from build123d import *

# Parameters (mm, degrees)
BASE_EXTRUDE_DEPTH = 11.1125
SKETCH2_R          = 4.1656
HOLE1_DEPTH        = 39.1
SKETCH3_R          = 3.2639
HOLE2_DEPTH        = 39.1


with BuildPart() as part:
    # Sketch1 → Base Extrude (new body, symmetric)
    with BuildSketch(Plane(origin=(0, 0, 0), x_dir=(0, 0, -1), z_dir=(1, 0, 0))):
        with BuildLine():
            Line((-4.7752, 9.5504), (-4.7752, 33.3248))
            ThreePointArc((-4.7752, 33.3248), (-3.376576302, 36.701376302), (0, 38.1))
            Line((0, 38.1), (0, 0))
            Line((0, 0), (-38.1, 0))
            ThreePointArc((-38.1, 0), (-36.701376302, 3.376576302), (-33.3248, 4.7752))
            Line((-33.3248, 4.7752), (-9.5504, 4.7752))
            ThreePointArc((-9.5504, 4.7752), (-6.173823698, 6.173823698), (-4.7752, 9.5504))
        make_face()
    extrude(amount=BASE_EXTRUDE_DEPTH, both=True)

    # Sketch2 → Hole1 (cut, through all)
    with BuildSketch(Plane.XZ):
        with Locations((0, 19.05)):
            Circle(SKETCH2_R)
    extrude(amount=-HOLE1_DEPTH, mode=Mode.SUBTRACT)

    # Sketch3 → Hole2 (cut, through all)
    with BuildSketch(Plane(origin=(0, 0, 0), x_dir=(-1, 0, 0), z_dir=(0, 0, -1))):
        with Locations((0, 19.05)):
            Circle(SKETCH3_R)
    extrude(amount=-HOLE2_DEPTH, mode=Mode.SUBTRACT)


solid = part.part
Geometry check sheet. Reference: the model listing, model coordinates, mm. A direction names the side the tool comes from. Give positions to 0.01 mm unless a question says otherwise; leave off trailing zeros. Write each loop counter-clockwise with the first axis right and the second up, starting at its lowest first coordinate (ties: lowest second). Pieces come first, ordered by that corner, then holes. Notation, with made-up numbers: M 88.5,30 L 93.5,30 A13 ccw 93.5,45 Z; hole C 46,-22.75 d4. An arc over 180 degrees is marked long. Answer as CSV lines item,"result". Start each with the question number.
Q1. Section check C-C, the plane z = 19.05. Record the cut outline in (x, y), then the cut area to 3 significant figures.
Q2. Section check B-B, the plane x = 0. Record the cut outline in (y, z).
Q3. Material ranges on L1, parallel to X at y = 2, z = 19; L2, parallel to X at y = 19, z = 3; L3, parallel to Y at x = 3.75, z = 24, recorded low to high.
Q4. Section check D-D, the plane x = 8.75. Record the cut outline in (y, z).
Q5. Section check A-A, the plane y = 19.05. Record the cut outline in (x, z), then the cut area to 3 significant figures.
Q6. Release check for a two-part mould opening along X. For faces 3 (the face through (-11.112, 7.9, 4.8)), 4 (the face through (-1.755, 21.802, 2.354)), 5 (the face through (0, 24, 0)) record: pulls with the +X half, pulls with the -X half, needs draft (parallel to the pull), parting line crosses it, or undercut.
Q7. Go/stop test with flat-tipped pins: pin 1 (2 mm diameter, centred on x = 0, y = 14, fed in from +Z); pin 2 (6.5 mm diameter, centred on x = -4, z = 23, fed in from +Y); pin 3 (4 mm diameter, centred on x = -6.5, z = 6, fed in from +Y). Record where each tip stops, or that it passes through.
Q8. Tool access check on faces 1 (the face through (-0.903, 2.354, 14.983)), 2 (the face through (0, 4.775, 24)). Record the directions out of +Z, -Z, +X, -X, +Y, -Y that give a thin tool (end or side, any length) a straight path to the whole face; none if there is none.
Geometry says:
1,outline,"M -11.11,0 L -4.17,0 L -4.17,4.78 L -11.11,4.78 Z; M 4.17,0 L 11.11,0 L 11.11,4.78 L 4.17,4.78 Z"
1,area,"66.3 mm^2"
2,outline,"M 0,0 L 15.79,0 L 15.79,4.78 L 9.55,4.78 A4.78 cw 4.78,9.55 L 4.78,14.88 L 0,14.88 Z; M 0,23.22 L 4.78,23.22 L 4.78,33.32 A4.78 ccw 0,38.1 Z; M 22.31,0 L 38.1,0 A4.78 ccw 33.32,4.78 L 22.31,4.78 Z"
3,L1,"-11.11 to -4.17, 4.17 to 11.11"
3,L2,"-11.11 to -3.26, 3.26 to 11.11"
3,L3,"0 to 4.78"
4,outline,"M 0,0 L 38.1,0 A4.78 ccw 33.32,4.78 L 9.55,4.78 A4.78 cw 4.78,9.55 L 4.78,33.32 A4.78 ccw 0,38.1 Z"
5,outline,"M -11.11,0 L -3.26,0 L -3.26,4.78 L -11.11,4.78 Z; M 3.26,0 L 11.11,0 L 11.11,4.78 L 3.26,4.78 Z"
5,area,"75.0 mm^2"
6,face 3,"pulls with the -X half"
6,face 4,"undercut"
6,face 5,"needs draft"
7,pin 1,"z = 4.78"
7,pin 2,"y = 4.78"
7,pin 3,"y = 35.93"
8,face 1,"+Y, -Y"
8,face 2,"+Z, +X, -X, +Y"
